from build123d import *

# Parameters (mm, degrees)
BOSS_EXTRUDE1_DEPTH = 202
CUT_EXTRUDE1_REACH  = 14
SKETCH2_R           = 2.25
CUT_EXTRUDE2_REACH  = 17
SKETCH3_R           = 2.25


with BuildPart() as part:
    # Sketch1 → Boss-Extrude1 (new body)
    with BuildSketch(Plane(origin=(0, 0, 0), x_dir=(1, 0, 0), z_dir=(0, 1, 0))):
        Polygon((0, 0), (15, 0), (15, 12), (14.5, 12), (14.5, 0.5), (0, 0.5), align=None)
    extrude(amount=BOSS_EXTRUDE1_DEPTH)

    # Sketch2 → Cut-Extrude1 (cut, up to next)
    with BuildSketch(Plane.XY, mode=Mode.PRIVATE) as cut_extrude1_sk1:
        with Locations((7.5, 175.166666667)):
            Circle(SKETCH2_R)
    cut_extrude1_tool1 = extrude(cut_extrude1_sk1.sketch, amount=-CUT_EXTRUDE1_REACH, mode=Mode.PRIVATE) & part.part
    add(cut_extrude1_tool1.solids().sort_by_distance((7.5, 175.166667, 0))[0], mode=Mode.SUBTRACT)
    # Sketch2 → Cut-Extrude1 (cut, up to next)
    with BuildSketch(Plane.XY, mode=Mode.PRIVATE) as cut_extrude1_sk2:
        with Locations((7.5, 141.833333333)):
            Circle(SKETCH2_R)
    cut_extrude1_tool2 = extrude(cut_extrude1_sk2.sketch, amount=-CUT_EXTRUDE1_REACH, mode=Mode.PRIVATE) & part.part
    add(cut_extrude1_tool2.solids().sort_by_distance((7.5, 141.833333, 0))[0], mode=Mode.SUBTRACT)
    # Sketch2 → Cut-Extrude1 (cut, up to next)
    with BuildSketch(Plane.XY, mode=Mode.PRIVATE) as cut_extrude1_sk3:
        with Locations((7.5, 108.5)):
            Circle(SKETCH2_R)
    cut_extrude1_tool3 = extrude(cut_extrude1_sk3.sketch, amount=-CUT_EXTRUDE1_REACH, mode=Mode.PRIVATE) & part.part
    add(cut_extrude1_tool3.solids().sort_by_distance((7.5, 108.5, 0))[0], mode=Mode.SUBTRACT)
    # Sketch2 → Cut-Extrude1 (cut, up to next)
    with BuildSketch(Plane.XY, mode=Mode.PRIVATE) as cut_extrude1_sk4:
        with Locations((7.5, 93.5)):
            Circle(SKETCH2_R)
    cut_extrude1_tool4 = extrude(cut_extrude1_sk4.sketch, amount=-CUT_EXTRUDE1_REACH, mode=Mode.PRIVATE) & part.part
    add(cut_extrude1_tool4.solids().sort_by_distance((7.5, 93.5, 0))[0], mode=Mode.SUBTRACT)
    # Sketch2 → Cut-Extrude1 (cut, up to next)
    with BuildSketch(Plane.XY, mode=Mode.PRIVATE) as cut_extrude1_sk5:
        with Locations((7.5, 60.166666667)):
            Circle(SKETCH2_R)
    cut_extrude1_tool5 = extrude(cut_extrude1_sk5.sketch, amount=-CUT_EXTRUDE1_REACH, mode=Mode.PRIVATE) & part.part
    add(cut_extrude1_tool5.solids().sort_by_distance((7.5, 60.166667, 0))[0], mode=Mode.SUBTRACT)
    # Sketch2 → Cut-Extrude1 (cut, up to next)
    with BuildSketch(Plane.XY, mode=Mode.PRIVATE) as cut_extrude1_sk6:
        with Locations((7.5, 26.833333333)):
            Circle(SKETCH2_R)
    cut_extrude1_tool6 = extrude(cut_extrude1_sk6.sketch, amount=-CUT_EXTRUDE1_REACH, mode=Mode.PRIVATE) & part.part
    add(cut_extrude1_tool6.solids().sort_by_distance((7.5, 26.833333, 0))[0], mode=Mode.SUBTRACT)

    # Sketch3 → Cut-Extrude2 (cut, up to next)
    with BuildSketch(Plane(origin=(15, 0, 0), x_dir=(0, 0, -1), z_dir=(1, 0, 0)), mode=Mode.PRIVATE) as cut_extrude2_sk1:
        with Locations((4.5, 24)):
            Circle(SKETCH3_R)
    cut_extrude2_tool1 = extrude(cut_extrude2_sk1.sketch, amount=-CUT_EXTRUDE2_REACH, mode=Mode.PRIVATE) & part.part
    add(cut_extrude2_tool1.solids().sort_by_distance((15, 24, -4.5))[0], mode=Mode.SUBTRACT)
    # Sketch3 → Cut-Extrude2 (cut, up to next)
    with BuildSketch(Plane(origin=(15, 0, 0), x_dir=(0, 0, -1), z_dir=(1, 0, 0)), mode=Mode.PRIVATE) as cut_extrude2_sk2:
        with Locations((4.5, 57.5)):
            Circle(SKETCH3_R)
    cut_extrude2_tool2 = extrude(cut_extrude2_sk2.sketch, amount=-CUT_EXTRUDE2_REACH, mode=Mode.PRIVATE) & part.part
    add(cut_extrude2_tool2.solids().sort_by_distance((15, 57.5, -4.5))[0], mode=Mode.SUBTRACT)
    # Sketch3 → Cut-Extrude2 (cut, up to next)
    with BuildSketch(Plane(origin=(15, 0, 0), x_dir=(0, 0, -1), z_dir=(1, 0, 0)), mode=Mode.PRIVATE) as cut_extrude2_sk3:
        with Locations((4.5, 91)):
            Circle(SKETCH3_R)
    cut_extrude2_tool3 = extrude(cut_extrude2_sk3.sketch, amount=-CUT_EXTRUDE2_REACH, mode=Mode.PRIVATE) & part.part
    add(cut_extrude2_tool3.solids().sort_by_distance((15, 91, -4.5))[0], mode=Mode.SUBTRACT)
    # Sketch3 → Cut-Extrude2 (cut, up to next)
    with BuildSketch(Plane(origin=(15, 0, 0), x_dir=(0, 0, -1), z_dir=(1, 0, 0)), mode=Mode.PRIVATE) as cut_extrude2_sk4:
        with Locations((4.5, 111)):
            Circle(SKETCH3_R)
    cut_extrude2_tool4 = extrude(cut_extrude2_sk4.sketch, amount=-CUT_EXTRUDE2_REACH, mode=Mode.PRIVATE) & part.part
    add(cut_extrude2_tool4.solids().sort_by_distance((15, 111, -4.5))[0], mode=Mode.SUBTRACT)
    # Sketch3 → Cut-Extrude2 (cut, up to next)
    with BuildSketch(Plane(origin=(15, 0, 0), x_dir=(0, 0, -1), z_dir=(1, 0, 0)), mode=Mode.PRIVATE) as cut_extrude2_sk5:
        with Locations((4.5, 144.5)):
            Circle(SKETCH3_R)
    cut_extrude2_tool5 = extrude(cut_extrude2_sk5.sketch, amount=-CUT_EXTRUDE2_REACH, mode=Mode.PRIVATE) & part.part
    add(cut_extrude2_tool5.solids().sort_by_distance((15, 144.5, -4.5))[0], mode=Mode.SUBTRACT)
    # Sketch3 → Cut-Extrude2 (cut, up to next)
    with BuildSketch(Plane(origin=(15, 0, 0), x_dir=(0, 0, -1), z_dir=(1, 0, 0)), mode=Mode.PRIVATE) as cut_extrude2_sk6:
        with Locations((4.5, 178)):
            Circle(SKETCH3_R)
    cut_extrude2_tool6 = extrude(cut_extrude2_sk6.sketch, amount=-CUT_EXTRUDE2_REACH, mode=Mode.PRIVATE) & part.part
    add(cut_extrude2_tool6.solids().sort_by_distance((15, 178, -4.5))[0], mode=Mode.SUBTRACT)


solid = part.part
Geometry check sheet. Reference: the model listing, model coordinates, mm. A direction names the side the tool comes from. Give positions to 0.01 mm unless a question says otherwise; leave off trailing zeros. Write each loop counter-clockwise with the first axis right and the second up, starting at its lowest first coordinate (ties: lowest second). Pieces come first, ordered by that corner, then holes. Notation, with made-up numbers: M 10.5,-3 L 67.5,-3 A20 cw 67.5,20 Z; hole C 58.5,70.5 d1. An arc over 180 degrees is marked long. Answer as CSV lines item,"result". Start each with the question number.
Q1. Material ranges on L1, parallel to X at y = 81, z = -9.5; L2, parallel to Z at x = 11, y = 172, recorded low to high.
Q2. Tool access check on faces 4 (the face through (7, 100, -0.5)), 5 (the face through (14.754, 108.804, -4.012)). Record the directions out of +Z, -Z, +X, -X, +Y, -Y that give a thin tool (end or side, any length) a straight path to the whole face; none if there is none.
Q3. Release check for a two-part mould opening along Y. For faces 1 (the face through (7.207, 144.064, -0.246)), 2 (the face through (7, 100, 0)), 3 (the face through (10.8, 202, -0.3)) record: pulls with the +Y half, pulls with the -Y half, needs draft (parallel to the pull), parting line crosses it, or undercut.
Q4. Section check A-A, the plane z = -4.5. Record the cut outline in (x, y).
Q5. Go/stop test with flat-tipped pins: pin 1 (7 mm diameter, centred on x = 7.5, y = 60.17, fed in from -Z); pin 2 (1.5 mm diameter, centred on y = 161.5, z = -5.5, fed in from -X). Record where each tip stops, or that it passes through.
Q6. Section check B-B, the plane x = 7.5. Record the cut outline in (y, z), then the cut area to 3 significant figures.
Q7. Section check C-C, the plane y = 66. Record the cut outline in (x, z).
Geometry says:
1,L1,"14.5 to 15"
1,L2,"-0.5 to 0"
2,face 4,"-Z, -X, +Y, -Y"
2,face 5,"+X, -X"
3,face 1,"undercut"
3,face 2,"needs draft"
3,face 3,"pulls with the +Y half"
4,outline,"M 14.5,0 L 15,0 L 15,21.75 L 14.5,21.75 Z; M 14.5,26.25 L 15,26.25 L 15,55.25 L 14.5,55.25 Z; M 14.5,59.75 L 15,59.75 L 15,88.75 L 14.5,88.75 Z; M 14.5,93.25 L 15,93.25 L 15,108.75 L 14.5,108.75 Z; M 14.5,113.25 L 15,113.25 L 15,142.25 L 14.5,142.25 Z; M 14.5,146.75 L 15,146.75 L 15,175.75 L 14.5,175.75 Z; M 14.5,180.25 L 15,180.25 L 15,202 L 14.5,202 Z"
5,pin 1,"z = -0.5"
5,pin 2,"x = 14.5"
6,outline,"M 0,-0.5 L 24.58,-0.5 L 24.58,0 L 0,0 Z; M 29.08,-0.5 L 57.92,-0.5 L 57.92,0 L 29.08,0 Z; M 62.42,-0.5 L 91.25,-0.5 L 91.25,0 L 62.42,0 Z; M 95.75,-0.5 L 106.25,-0.5 L 106.25,0 L 95.75,0 Z; M 110.75,-0.5 L 139.58,-0.5 L 139.58,0 L 110.75,0 Z; M 144.08,-0.5 L 172.92,-0.5 L 172.92,0 L 144.08,0 Z; M 177.42,-0.5 L 202,-0.5 L 202,0 L 177.42,0 Z"
6,area,"87.5 mm^2"
7,outline,"M 0,-0.5 L 14.5,-0.5 L 14.5,-12 L 15,-12 L 15,0 L 0,0 Z"
